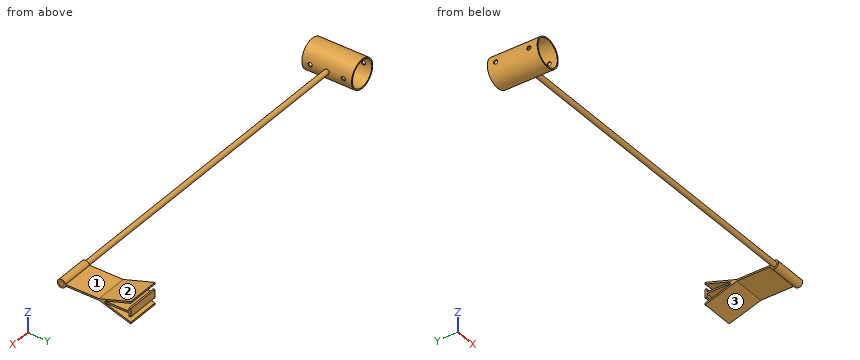
Autodesk Inventor part; units mm, degrees
ref_plane "YZ Plane" through (0, 0, 0) normal (1, 0, 0) x (0, 1, 0)
ref_plane "XZ Plane" through (0, 0, 0) normal (0, 1, 0) x (-1, 0, 0)
ref_plane "XY Plane" through (0, 0, 0) normal (0, 0, 1) x (1, 0, 0)
sketch "Esboço1" plane through (0, 0, 0) normal (0, 1, 0) x (-1, 0, 0)
  circle A0 centre (0, 0) radius 16
  circle A1 centre (0, 0) radius 17.5
  dimension "d0" = 32
  dimension "d1" = 35
extrude "Extrusão1" add sketch "Esboço1" along normal mid plane 60
sketch "Esboço2" plane through (0, 0, 0) normal (0, 1, 0) x (-1, 0, 0)
  circle A0 centre (0, 0) radius 17.5
  line L0 (-17.5, 0) -> (-417.5, 0)
  line L1 (-417.5, 0) -> (-417.5, 3)
  circle A1 centre (0, 0) radius 9.5
  line L2 (-26.4835, 0) -> (-26.4835, 3)
  line L3 (-17.2409, 3) -> (-417.5, 3)
  point P0 (-15.8635, 7.3891)
  dimension "d4" = 400
  dimension "d5" = 3
  dimension "d6" = 19
  dimension "d60" = 3
revolve "Revolução1" add sketch "Esboço2" angle 360 about axis through (17.5, 0, 0) along (1, 0, 0) contours A0 L0 L2 L3 | L2 L0 L1 L3
sketch "Esboço3" plane through (0, 0, 0) normal (0, 1, 0) x (-1, 0, 0)
  line L0 (-417.5, -3) -> (-417.5, 3)
  line L1 (-417.5, 0) -> (-417.5, 15)
  line L2 (-417.5, 15) -> (-417.5, -15)
  line L3 (-417.5, -15) -> (-457.5, -15)
  line L4 (-457.5, -15) -> (-457.5, 15)
  line L5 (-457.5, 15) -> (-417.5, 15)
  point P0 (0, 0)
  dimension "d8" = 15
  dimension "d9" = 30
  dimension "d10" = 40
extrude "Extrusão2" add sketch "Esboço3" along normal mid plane 170
sketch "Esboço5" plane through (457.5, -85, -15) normal (1, 0, 0) x (0, 0, -1)
  circle A0 centre (-15, 85) radius 4
  circle A1 centre (-15, 85) radius 3
  line L0 (-16.25, 88.0318) -> (-14.25, 88.0318)
  line L1 (-14.25, 88.0318) -> (-14.25, 87.9047)
  line L2 (-14.25, 87.9047) -> (0, 87.9047)
  line L3 (0, 0) -> (0, 170)
  line L4 (-15.75, 87.9047) -> (-30, 87.9047)
  line L5 (-30, 170) -> (-30, 0)
  line L6 (-30, 87.9047) -> (-30, 0)
  line L7 (0, 0) -> (-30, 0)
  line L8 (-30, 0) -> (0, 0)
  line L9 (0, 0) -> (0, 87.9047)
  circle A2 centre (-15, 85) radius 5
  line L10 (-15.9946, 130.4066) -> (-13.9946, 130.4094)
  line L11 (-13.9946, 130.4094) -> (-14.0909, 89.9167)
  line L12 (-15.9946, 130.4066) -> (-28.3553, 168.4488)
  line L13 (-15.9946, 130.4066) -> (24.0054, 130.4066) construction
  line L14 (-13.9946, 130.4094) -> (-1.6339, 168.4517)
  line L15 (-13.9946, 130.4094) -> (26.0054, 130.4094) construction
  line L16 (-18.099, 136.8832) -> (-16.1969, 137.5013)
  line L17 (-25.4193, 159.413) -> (-23.5172, 160.031)
  line L18 (-4.4713, 159.7191) -> (-6.3734, 160.3371)
  line L19 (-10.3922, 141.4965) -> (-12.2943, 142.1146)
  line L20 (-28.3553, 168.4488) -> (-26.2523, 168.4488)
  line L21 (-1.6339, 168.4517) -> (-3.7368, 168.4517)
  line L22 (-15.0524, 134.2763) -> (-15.0666, 134.2336)
  line L23 (-15.9946, 168.4488) -> (-13.9946, 168.4488)
  line L24 (-15.9946, 89.9001) -> (-15.9946, 130.4066)
  line L25 (-15.9946, 136.8787) -> (-15.9946, 168.4488)
  line L26 (-13.9946, 168.4488) -> (-13.9946, 136.8787)
  line L27 (-15.9946, 136.8787) -> (-26.2523, 168.4488)
  line L28 (-13.9946, 136.8787) -> (-3.7368, 168.4517)
  line L29 (-15.9946, 168.4488) -> (-19.9946, 168.4488)
  line L30 (-19.9946, 168.4488) -> (-9.9946, 168.4488)
  line L31 (-9.9946, 168.4488) -> (-9.9946, 166.4488)
  line L32 (-9.9946, 166.4488) -> (-19.9946, 166.4488)
  line L33 (-19.9946, 166.4488) -> (-19.9946, 168.4488)
  line L34 (-15.9946, 168.4488) -> (-15.9946, 156.4488)
  line L35 (-15.9946, 156.4488) -> (-18.9946, 156.4488)
  line L36 (-18.9946, 156.4488) -> (-18.9946, 146.4488)
  line L37 (-18.9946, 146.4488) -> (-15.9946, 146.4488)
  line L38 (-13.9946, 156.4488) -> (-10.9946, 156.4488)
  line L39 (-10.9946, 156.4488) -> (-10.9946, 146.4488)
  line L40 (-10.9946, 146.4488) -> (-13.9946, 146.4488)
  line L41 (-30, 170) -> (0, 170)
  line L42 (-30, 170) -> (-30, 0)
  line L43 (0, 0) -> (0, 170)
  line L44 (0, 0) -> (-30, 0)
  line L45 (0, 0) -> (0, 170)
  line L46 (-30, 170) -> (0, 170)
  point P0 (-15, 85)
  point P1 (-15.9946, 166.4488)
  point P2 (-13.9946, 166.4488)
  dimension "d15" = 10
  dimension "d17" = 2
  dimension "d19" = 40
  dimension "d20" = 108
  dimension "d21" = 40
  dimension "d22" = 72
  dimension "d23" = 2
  dimension "d24" = 2
  dimension "d25" = 2
  dimension "d26" = 2
  dimension "d29" = 36
  dimension "d31" = 2
  dimension "d34" = 4
  dimension "d35" = 10
  dimension "d36" = 2
  dimension "d37" = 12
  dimension "d38" = 3
  dimension "d39" = 10
  dimension "d40" = 3
  dimension "d42" = 10
extrude "Extrusão3" cut sketch "Esboço5" against normal blind 170 contours A2 L11 L14 L21 L28 L26 L40 L39 L38 L32 L31 L30 L23 L29 L33 L25 L35 L36 L37 L27 L20 L12 L24 L4 L5 L41 L3 L2 | L2 L3 L7 L5 L4 A2
sketch "Esboço6" plane through (457.5, 4.9001, 0.9946) normal (1, 0, 0) x (0, 0, -1)
  circle A0 centre (0.9946, -4.9001) radius 3
  dimension "d61" = 6
extrude "Extrusão4" cut sketch "Esboço6" against normal blind 0.01
sketch "Esboço7" plane through (457.5, 4.9001, 0.9946) normal (1, 0, 0) x (0, 0, -1)
  line L0 (0, 66.5487) -> (-3, 66.5487)
  line L1 (-3, 56.5487) -> (0, 56.5487)
  line L2 (0, 66.5487) -> (0, 56.5487)
  line L3 (0, 56.5487) -> (-3, 56.5487)
  line L4 (-3, 66.5487) -> (-3, 56.5487)
  line L5 (-3, 56.5487) -> (-3, 66.5487)
  line L6 (-3, 66.5487) -> (0, 66.5487)
  line L7 (2, 56.5487) -> (5, 56.5487)
  line L8 (2, 56.5487) -> (5, 56.5487)
  line L9 (2, 66.5487) -> (5, 66.5487)
  line L10 (5, 56.5487) -> (5, 66.5487)
  line L11 (5, 66.5487) -> (2, 66.5487)
  line L12 (2, 66.5487) -> (2, 56.5487)
  point P0 (0.9946, -4.9001)
extrude "Extrusão5" cut sketch "Esboço7" against normal blind 10
sketch "Esboço8" plane through (417.5, 4.9001, 0.9946) normal (-1, 0, 0) x (0, 0, 1)
  line L0 (-2, 76.5487) -> (-2, 66.5487)
  line L1 (-2, 56.5487) -> (-2, 46.9786)
  line L2 (-2, 66.5487) -> (-2, 56.5487)
  line L3 (-5, 56.5487) -> (-2, 56.5487)
  line L4 (-2, 56.5487) -> (-5, 56.5487)
  line L5 (-5, 56.5487) -> (-5, 66.5487)
  line L6 (-5, 66.5487) -> (-2, 66.5487)
  line L7 (3, 66.5487) -> (0, 66.5487)
  line L8 (0, 66.5487) -> (3, 66.5487)
  line L9 (3, 66.5487) -> (3, 56.5487)
  line L10 (0, 46.9786) -> (0, 56.5487)
  line L11 (3, 56.5487) -> (0, 56.5487)
  line L12 (0, 56.5487) -> (0, 66.5487)
  line L13 (0, 76.5487) -> (0, 46.9786)
  point P0 (-0.9946, -4.9001)
extrude "Extrusão6" cut sketch "Esboço8" against normal blind 15
fillet "Arredondamento1" radius 5 4 edges at (447.5, 71.4488, 2.4946) (447.5, 61.4488, 2.4946) (447.5, 61.4488, -2.5054) (447.5, 71.4488, -2.5054)
sketch "Esboço9" plane through (0, 0, 0) normal (1, 0, 0) x (0, 1, 0)
  line L0 (30, -17.5) -> (30, 17.5)
  line L1 (30, 0) -> (20, 0)
  line L2 (-30, -16) -> (-30, 16)
  line L3 (-30, 0) -> (-20, 0)
  circle A0 centre (20, 0) radius 2.5
  circle A1 centre (-20, 0) radius 2.5
  point P0 (0, 0)
  dimension "d52" = 10
  dimension "d53" = 10
  dimension "d56" = 5
  dimension "d57" = 5
extrude "Extrusão7" cut sketch "Esboço9" along normal mid plane 150
properties part number "LDR"
The listing builds one solid part. Answer for the finished solid, in the listing's coordinates (mm). Face numbers are marked on the shaded views. A direction names the side the tool comes from. Round coordinates to 2 decimals unless told otherwise and drop trailing zeros. Order: outer loops, then holes, each group sorted by start corner. A loop starts at its lowest first (then second) coordinate and runs counter-clockwise, first axis right, second up. Notation, with made-up numbers: M 22,51 L 70,51 A34 cw 70,83 Z; hole C -5.75,-37.5 d5. An arc over 180 degrees is marked long. Answer in a Markdown table with one row per item. Add a question column.
1) The part is cut by section C-C on x = 180. Determine the outline of the cut face in (y, z).
2) The part is cut by section B-B on y = 11. Determine the outline of the cut face in (x, z).
3) The part is cut by section A-A on x = 0. Determine the outline of the cut face in (y, z), plus the area to 3 significant figures.
4) Flat-ended cylindrical pins translate along their axes: pin 1 Ø4.5 at (x, z) = (435.5, -2.5) entering from -Y; pin 2 Ø1.5 at (y, z) = (65, -2) entering from -X; pin 3 Ø11 at (x, y) = (443.5, 68) entering from +Z; pin 4 Ø19 at (x, z) = (0, 0) entering from +Y (1 decimal). Find the tip coordinate at first contact, or state that the pin passes through.
5) Which of the six approach directions +Z, -Z, +X, -X, +Y, -Y give full straight-line access (tool end or side, diameter ignored) to the marked faces 1, 2 and 3?
6) Consider line 1 along X through (y, z) = (16.5, 0); line 2 along X through (y, z) = (12, 1.5); line 3 along X through (y, z) = (-2.5, 4). Determine where each line is inside the solid, lowest interval first. Write a range as from..to.
Findings below:
| question | item | result |
|---|---|---|
| 1 | outline | C 0,0 d6 |
| 2 | outline | C 0,0 d35; M 417.5,-0.92 L 457.5,-0.92 L 457.5,0.99 L 417.5,0.99 Z; hole C 0,0 d32 |
| 3 | outline | M -30,-17.5 L 30,-17.5 L 30,-16 L -30,-16 Z; M -30,16 L 30,16 L 30,17.5 L -30,17.5 Z |
| 3 | area | 180 mm² |
| 4 | pin 1 | stops at y = -4.99 |
| 4 | pin 2 | stops at x = 432.5 |
| 4 | pin 3 | stops at z = 10.12 |
| 4 | pin 4 | passes through |
| 5 | face 1 | +Z, +X |
| 5 | face 2 | +Z, +X, -X |
| 5 | face 3 | -Z, +X, -X |
| 6 | line 1 | x = -17.5..-16, 16..17.5, 417.5..457.5 |
| 6 | line 2 | x = -17.44..-15.93, 15.93..17.44 |
| 6 | line 3 | x = -17.04..-15.49, 15.49..17.04, 417.5..457.5 |
